```python
from build123d import *

# Parameters (mm, degrees)
SKETCH1_W           = 189.477532672
SKETCH1_H           = 19.05
BOSS_EXTRUDE1_DEPTH = 60.325
HOLE1_D             = 3.175
HOLE1_DEPTH         = 38.1
HOLE1_CSINK_D       = 10.16
HOLE1_CSINK_ANGLE   = 82
HOLE1_TIP           = 0.953866233


with BuildPart() as part:
    # Sketch1 → Boss-Extrude1 (new body)
    with BuildSketch(Plane.XY):
        with Locations((228.6, -9.525)):
            Rectangle(SKETCH1_W, SKETCH1_H)
    extrude(amount=BOSS_EXTRUDE1_DEPTH)

    # Hole1
    with Locations(Plane(origin=(228.6, 0, -25.4), x_dir=(-1, 0, 0), z_dir=(0, 0, -1))):
        with Locations((-75.688766336, -9.525), (218.563766336, -31.75), (218.563766336, -218.821), (218.563766336, -418.592), (104.263766336, -19.05), (104.263766336, -149.225), (104.263766336, -279.4), (120.138766336, -330.2), (120.138766336, -441.325), (-120.138766336, -441.325), (-120.138766336, -330.2), (-104.263766336, -279.4), (-104.263766336, -149.225), (-104.263766336, -19.05), (-218.563766336, -418.592), (-218.563766336, -218.821), (-218.563766336, -31.75), (0, -304.8), (107.438766336, -304.8), (-107.438766336, -304.8), (75.688766336, -276.225), (0, -276.225), (-75.688766336, -276.225), (75.688766336, -9.525), (0, -9.525)):
            CounterSinkHole(HOLE1_D / 2, HOLE1_CSINK_D / 2, depth=HOLE1_DEPTH, counter_sink_angle=HOLE1_CSINK_ANGLE)
            with Locations((0, 0, -(HOLE1_DEPTH + HOLE1_TIP / 2))):  # 118° drill point
                Cone(0, HOLE1_D / 2, HOLE1_TIP, mode=Mode.SUBTRACT)


solid = part.part
```
Can you work these out from the model? Positions are in its coordinate system, mm. A direction names the side the tool comes from. Give positions to 0.01 mm unless a question says otherwise; leave off trailing zeros. Answer in a Markdown table with one row per item.
1. If I drill on line 1 along Y through (x, z) = (228.6, 5.25); line 2 along Z through (x, y) = (154, -8.75) (3 decimals), over which ranges is the centre line in solid material (lowest first)?
Taken from the geometry:
| item | result |
|---|---|
| line 1 | y = -19.05 to -11.11, -7.94 to 0 |
| line 2 | z = 12.851 to 60.325 |
2. Thinking about a two-plate mould opening in Y: for faces 3 (the cylindrical face through (305.803, -9.048, 6.439)), 4 (the flat face through (227, 0, 30)), 5 (the flat face through (227, -9, 60.325)), which applies, released by +Y, released by -Y, zero draft, split by the parting line, or undercut?
Taken from the geometry:
| item | result |
|---|---|
| face 3 | undercut |
| face 4 | released by +Y |
| face 5 | zero draft |
3. Which directions (+Z, -Z, +X, -X, +Y, -Y) give clear straight access to the entire face, cutting with the end or side of a thin tool? Please do faces 1 (the cylindrical face through (230.1, -9, 6.4)), 2 (the flat face through (133.861, -10, 30)).
Taken from the geometry:
| item | result |
|---|---|
| face 1 | -Z |
| face 2 | +Z, -Z, -X, +Y, -Y |
